Design review of the part built by this model. Coordinates are the model's own, in mm. Round coordinates to 2 decimals unless told otherwise and drop trailing zeros. Loops run counter-clockwise (first coordinate to the right, second up) from the corner with the lowest first, then second, coordinate; pieces in that order, holes last. Notation, with made-up numbers: (-32.5, -9.75) - (-15.5, -9.75) arc R17 cw to (-15.5, 21.25) - close; hole circle Ø8 at (35.5, 3). An arc over 180 degrees is marked (long way). Return JSON: item names as keys, results as strings. Group by question number.
(1) We need section B-B, the plane y = 1.7. Give the number of separate pieces and of enclosed holes in the cut face, and give its area (3 significant figures).
(2) Wall thickness on L1, parallel to Z at x = 58, y = 5.75; L2, parallel to Z at x = -138, y = 1.35: over which ranges is each line inside the solid? List them lowest first. Write a range as [from, to].
(3) We need section A-A, the plane x = -6.5. Write out the cut boundary in (y, z), and give its area (3 significant figures).
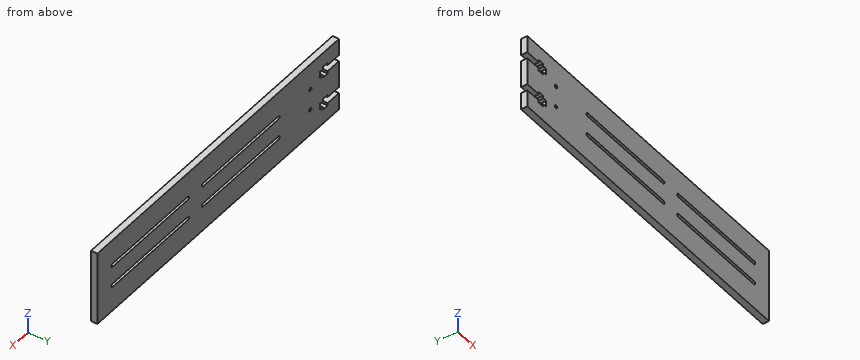
from build123d import *

# Parameters (mm, degrees)
SKETCH1_W           = 320
SKETCH1_H           = 70
BOSS_EXTRUDE1_DEPTH = 6
CUT_EXTRUDE2_DEPTH  = 7
CUT_EXTRUDE3_DEPTH  = 7
SKETCH6_R           = 1.6
CUT_EXTRUDE4_DEPTH  = 7


with BuildPart() as part:
    # Sketch1 → Boss-Extrude1 (new body)
    with BuildSketch(Plane(origin=(0, 0, 0), x_dir=(1, 0, 0), z_dir=(0, 1, 0))):
        Rectangle(SKETCH1_W, SKETCH1_H)
    extrude(amount=BOSS_EXTRUDE1_DEPTH)

    # Sketch3 → Cut-Extrude2 (cut, through all)
    with BuildSketch(Plane(origin=(0, 6, 0), x_dir=(1, 0, 0), z_dir=(0, 1, 0))):
        Polygon((-160, 12.9), (-145, 12.9), (-145, 10.5), (-139, 10.5), (-139, 12.9), (-135, 12.9), (-135, 18.9), (-139, 18.9), (-139, 21.3), (-145, 21.3), (-145, 18.9), (-160, 18.9), align=None)
        Polygon((-145, -18.9), (-145, -21.3), (-139, -21.3), (-139, -18.9), (-135, -18.9), (-135, -12.9), (-139, -12.9), (-139, -10.5), (-145, -10.5), (-145, -12.9), (-160, -12.9), (-160, -18.9), align=None)
    extrude(amount=-CUT_EXTRUDE2_DEPTH, mode=Mode.SUBTRACT)

    # Sketch5 → Cut-Extrude3 (cut, through all)
    with BuildSketch(Plane(origin=(0, 6, 0), x_dir=(1, 0, 0), z_dir=(0, 1, 0))):
        with BuildLine():
            Line((40, -8.4), (140, -8.4))
            ThreePointArc((140, -8.4), (141.6, -10), (140, -11.6))
            Line((140, -11.6), (40, -11.6))
            ThreePointArc((40, -11.6), (38.4, -10), (40, -8.4))
        make_face()
        with BuildLine():
            Line((-80, -8.4), (20, -8.4))
            ThreePointArc((20, -8.4), (21.6, -10), (20, -11.6))
            Line((20, -11.6), (-80, -11.6))
            ThreePointArc((-80, -11.6), (-81.6, -10), (-80, -8.4))
        make_face()
        with BuildLine():
            Line((-80, 11.6), (20, 11.6))
            ThreePointArc((20, 11.6), (21.6, 10), (20, 8.4))
            Line((20, 8.4), (-80, 8.4))
            ThreePointArc((-80, 8.4), (-81.6, 10), (-80, 11.6))
        make_face()
        with BuildLine():
            Line((40, 11.6), (140, 11.6))
            ThreePointArc((140, 11.6), (141.6, 10), (140, 8.4))
            Line((140, 8.4), (40, 8.4))
            ThreePointArc((40, 8.4), (38.4, 10), (40, 11.6))
        make_face()
    extrude(amount=-CUT_EXTRUDE3_DEPTH, mode=Mode.SUBTRACT)

    # Sketch6 → Cut-Extrude4 (cut, through all)
    with BuildSketch(Plane.XZ):
        with Locations((-122, -10)):
            Circle(SKETCH6_R)
        with Locations((-122, 10)):
            Circle(SKETCH6_R)
    extrude(amount=-CUT_EXTRUDE4_DEPTH, mode=Mode.SUBTRACT)


solid = part.part
Solutions:
{
 "1": {"separate pieces": "1", "enclosed holes": "6", "area": "20,700 mm^2"},
 "2": {"L1": "[-35, -11.6], [-8.4, 8.4], [11.6, 35]", "L2": "[-35, -18.9], [-12.9, 12.9], [18.9, 35]"},
 "3": {"outline": "(0, -35) - (6, -35) - (6, -11.6) - (0, -11.6) - close; (0, -8.4) - (6, -8.4) - (6, 8.4) - (0, 8.4) - close; (0, 11.6) - (6, 11.6) - (6, 35) - (0, 35) - close", "area": "382 mm^2"}
}
